from build123d import *

# Parameters (mm, degrees)
F0_W     = 84.3636319041
F0_H     = 35.2298701182
F1_DEPTH = 25.4
F2_R     = 6.3162901038
F3_DEPTH = 25.401
F4_R     = 6.4811389114
F5_DEPTH = 84.3646319041


with BuildPart() as f1:
    # F0 (on Front) → F1 (new body)
    with BuildSketch(Plane.XZ):
        with Locations((-0.2784244716, 2.2862604819)):
            Rectangle(F0_W, F0_H)
    extrude(amount=F1_DEPTH)

    # F2 (on face) → F3 (cut, through all)
    with BuildSketch(Plane.XZ.offset(25.4)):
        Circle(F2_R)
    extrude(amount=-F3_DEPTH, mode=Mode.SUBTRACT)

    # F4 (on face) → F5 (cut, through all)
    with BuildSketch(Plane.YZ.offset(41.9033914804)):
        with Locations((-12.7, 0)):
            Circle(F4_R)
    extrude(amount=-F5_DEPTH, mode=Mode.SUBTRACT)


solid = f1.part
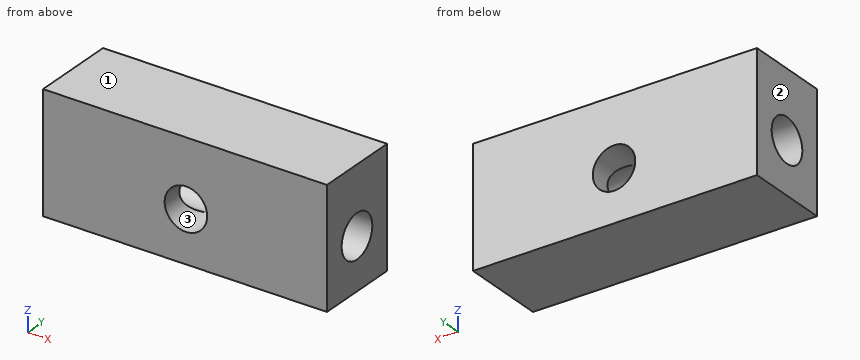
The listing builds one solid part. Answer for the finished solid, in the listing's coordinates (mm). Face numbers are marked on the shaded views. Coordinates: 2 decimals unless noted, no trailing zeros. Loops run counter-clockwise (first coordinate to the right, second up) from the corner with the lowest first, then second, coordinate; pieces in that order, holes last.
1) Determine the mould class of the marked faces 1, 2 and 3 for opening direction X: pulls with the +X half, pulls with the -X half, needs draft (parallel to the pull), parting line crosses it, or undercut.
2) A flat-ended cylindrical pin translates along its axis: pin 1 Ø20 at (x, z) = (0, 0) entering from +Y. Find the tip coordinate at first contact, or state that the pin passes through.
3) Find section B-B on y = -12.7. Write down the section's boundary in (x, z).
4) Find the intervals of material crossed by L1, parallel to Z at x = -3.5, y = -12.7; L2, parallel to X at y = -22.5, z = 0; L3, parallel to Z at x = 0, y = -8.5, in increasing order.
5) Find section C-C on x = 0. Write down the section's boundary in (y, z).
6) Find section D-D on y = -5.25. Write down the section's boundary in (x, z).
7) Find section A-A on z = 0. Write down the section's boundary in (x, y).
Values:
1. face 1: needs draft
1. face 2: pulls with the -X half
1. face 3: undercut
2. pin 1: stops at y = 0
3. outline: (-42.46, -15.33) - (41.9, -15.33) - (41.9, -6.48) - (-42.46, -6.48) - close; (-42.46, 6.48) - (41.9, 6.48) - (41.9, 19.9) - (-42.46, 19.9) - close
4. L1: z = -15.33 to -6.48, 6.48 to 19.9
4. L2: x = -42.46 to -6.32, 6.32 to 41.9
4. L3: z = -15.33 to -6.32, 6.32 to 19.9
5. outline: (-25.4, -15.33) - (0, -15.33) - (0, -6.32) - (-11.25, -6.32) arc R6.48 cw to (-14.15, -6.32) - (-25.4, -6.32) - close; (-25.4, 6.32) - (-14.15, 6.32) arc R6.48 cw to (-11.25, 6.32) - (0, 6.32) - (0, 19.9) - (-25.4, 19.9) - close
6. outline: (-42.46, -15.33) - (41.9, -15.33) - (41.9, 19.9) - (-42.46, 19.9) - close; hole circle Ø12.63 at (0, 0)
7. outline: (-42.46, -25.4) - (-6.32, -25.4) - (-6.32, -19.18) - (-42.46, -19.18) - close; (-42.46, -6.22) - (-6.32, -6.22) - (-6.32, 0) - (-42.46, 0) - close; (6.32, -25.4) - (41.9, -25.4) - (41.9, -19.18) - (6.32, -19.18) - close; (6.32, -6.22) - (41.9, -6.22) - (41.9, 0) - (6.32, 0) - close
